Autodesk Inventor part; units mm, degrees
ref_plane "YZ Plane" through (0, 0, 0) normal (1, 0, 0) x (0, 1, 0)
ref_plane "XZ Plane" through (0, 0, 0) normal (0, 1, 0) x (-1, 0, 0)
ref_plane "XY Plane" through (0, 0, 0) normal (0, 0, 1) x (1, 0, 0)
sketch "Sketch1" plane through (0, 0, 0) normal (0, 0, 1) x (1, 0, 0)
  arc A0 (-13.7715, -6.45) -> (-16.2715, -6.45) centre (-15.0215, -6.45) ccw
  line L0 (-16.2715, -6.45) -> (-16.2715, -7.25)
  arc A1 (-17.2715, -8.25) -> (-16.2715, -7.25) centre (-17.2715, -7.25) ccw
  line L1 (-17.2715, -8.25) -> (-18.7715, -8.25)
  arc A2 (-19.7715, -7.25) -> (-18.7715, -8.25) centre (-18.7715, -7.25) ccw
  line L2 (-19.7715, -7.25) -> (-19.7715, 7.25)
  arc A3 (-18.7715, 8.25) -> (-19.7715, 7.25) centre (-18.7715, 7.25) ccw
  line L3 (-18.7715, 8.25) -> (-17.2715, 8.25)
  arc A4 (-16.2715, 7.25) -> (-17.2715, 8.25) centre (-17.2715, 7.25) ccw
  line L4 (-16.2715, 7.25) -> (-16.2715, 6.45)
  arc A5 (-16.2715, 6.45) -> (-13.7715, 6.45) centre (-15.0215, 6.45) ccw
  arc A6 (-13.5715, -6.45) -> (-16.4715, -6.45) centre (-15.0215, -6.45) ccw
  line L5 (-16.4715, -6.45) -> (-16.4715, -7.25)
  arc A7 (-17.2715, -8.05) -> (-16.4715, -7.25) centre (-17.2715, -7.25) ccw
  line L6 (-17.2715, -8.05) -> (-18.7715, -8.05)
  arc A8 (-19.5715, -7.25) -> (-18.7715, -8.05) centre (-18.7715, -7.25) ccw
  line L7 (-19.5715, -7.25) -> (-19.5715, 7.25)
  arc A9 (-18.7715, 8.05) -> (-19.5715, 7.25) centre (-18.7715, 7.25) ccw
  line L8 (-18.7715, 8.05) -> (-17.2715, 8.05)
  arc A10 (-16.4715, 7.25) -> (-17.2715, 8.05) centre (-17.2715, 7.25) ccw
  line L9 (-16.4715, 7.25) -> (-16.4715, 6.45)
  arc A11 (-16.4715, 6.45) -> (-13.5715, 6.45) centre (-15.0215, 6.45) ccw
  circle A12 centre (-5.5215, 0) radius 1.6
  circle A13 centre (7.4785, 5) radius 0.5969
  circle A14 centre (7.4785, -5) radius 0.5969
  line L10 (13.4965, -5.336) -> (13.0086, -5.8402)
  arc A15 (13.4965, -5.336) -> (1.4605, 5.336) centre (7.4785, 0) ccw
  line L11 (1.1785, 5) -> (1.4605, 5.336)
  line L12 (-15.5215, 5) -> (1.1785, 5)
  line L13 (-15.5215, -5) -> (-15.5215, 5)
  line L14 (1.1785, -5) -> (-15.5215, -5)
  arc A16 (1.1785, -5) -> (13.0086, -5.8402) centre (7.4785, 0) ccw
  arc A17 (-0.6485, -6.45) -> (-0.6486, 6.45) centre (7.4785, 0) ccw
  line L15 (-0.6485, -6.45) -> (-15.5215, -6.45)
  line L16 (-15.5215, -6.45) -> (-15.5215, 6.45)
  line L17 (-15.5215, 6.45) -> (-0.6486, 6.45)
  line L18 (7.4785, 0) -> (-0.6485, -6.45)
  line L19 (7.4785, 0) -> (-0.6486, 6.45)
  circle A18 centre (7.4785, 0) radius 8.243
  point P0 (0, 0)
  point P1 (-15.03, 5)
  point P2 (-15.5215, 5.0889)
  point P3 (-13.5715, 6.45)
  dimension "d0" = 0.2
  dimension "d1" = 0.2
extrude "Extrusion1" add sketch "Sketch1" against normal blind 10 contours A6 L14 A18 L18 L15 | L16 L14 A6 | A6 L5 A7 L6 A8 L7 A9 L8 A10 L9 A11 L16 L13 | L14 L13 L12 A18 | L18 A18 L19 A17 | L19 A18 L12 A11 L17 | A12
sketch "Sketch2" plane through (0, 0, 0) normal (0, 0, 1) x (1, 0, 0)
  circle A0 centre (-5.5215, 0) radius 1.6
  circle A1 centre (7.4785, 5) radius 0.5969
  circle A2 centre (7.4785, -5) radius 0.5969
  line L0 (13.4965, -5.336) -> (13.0086, -5.8402)
  arc A3 (13.4965, -5.336) -> (1.4605, 5.336) centre (7.4785, 0) ccw
  line L1 (1.1785, 5) -> (1.4605, 5.336)
  line L2 (-15.5215, 5) -> (1.1785, 5)
  line L3 (-15.5215, -5) -> (-15.5215, 5)
  line L4 (1.1785, -5) -> (-15.5215, -5)
  arc A4 (1.1785, -5) -> (13.0086, -5.8402) centre (7.4785, 0) ccw
  line L5 (-15.7215, 5.2) -> (1.0853, 5.2)
  line L6 (1.0853, 5.2) -> (1.309, 5.4667)
  arc A5 (13.6433, -5.472) -> (1.309, 5.4667) centre (7.4785, 0) ccw
  line L7 (13.6433, -5.472) -> (13.1493, -5.9824)
  arc A6 (1.0826, -5.2) -> (13.1493, -5.9824) centre (7.4785, 0) ccw
  line L8 (1.0826, -5.2) -> (-15.7215, -5.2)
  line L9 (-15.7215, -5.2) -> (-15.7215, 5.2)
  point P0 (0, 0)
  dimension "d4" = 0.2
extrude "Extrusion2" cut sketch "Sketch2" against normal blind 1.6 contours L0 A4 L4 L3 L2 L1 A3 | L5 L6 A5 L7 A6 L8 L9
sketch "Sketch3" plane through (-5.5215, 0, 0) normal (0, 0, 1) x (1, 0, 0)
  circle A0 centre (0, 0) radius 2
  point P0 (5.5215, 0)
  dimension "d7" = 4
extrude "Extrusion3" cut sketch "Sketch3" against normal blind 8
sketch "Sketch4" plane through (-19.5715, -7.25, 0) normal (-1, 0, 0) x (0, 0, 1)
  circle A0 centre (-5, 7.25) radius 2
  point P0 (0, 7.25)
  dimension "d10" = 4
  dimension "d11" = 5
extrude "Extrusion4" cut sketch "Sketch4" against normal blind 8
sketch "Sketch5" plane through (0, 0, 0) normal (0, 0, 1) x (1, 0, 0)
  line L0 (-13.7715, -9.5) -> (-13.7715, -6.45)
  line L1 (-13.7715, 6.45) -> (-13.7715, 9.5)
  line L2 (-13.7715, -9.5) -> (3.307, -9.5)
  arc A0 (-0.6485, -6.45) -> (-0.6486, 6.45) centre (7.4785, 0) ccw
  line L3 (-13.7715, 9.5) -> (3.307, 9.5)
  line L4 (-0.6485, -6.45) -> (-13.5715, -6.45)
  line L5 (-13.5715, -6.45) -> (-13.5715, -9.5)
  arc A1 (-15.03, 5) -> (-13.5715, 6.45) centre (-15.0215, 6.45) ccw
  line L6 (-13.5715, 6.45) -> (-13.5715, 9.5)
  line L7 (-0.6486, 6.45) -> (-13.5715, 6.45)
  point P0 (0, 0)
extrude "Extrusion5" add sketch "Sketch5" against normal up to surface (10 mm away)
fillet "Fillet2" radius 1 6 edges at (17.854, 0, 0) (-5.1322, -9.5, 0) (-5.1323, 9.5, 0) (17.854, 0, -10) (-5.1323, 9.5, -10) (-5.1322, -9.5, -10)
properties part number "TransducerPCB_Holder"
The listing builds one solid part. Answer for the finished solid, in the listing's coordinates (mm). A direction names the side the tool comes from. Give positions to 0.01 mm unless a question says otherwise; leave off trailing zeros. Loops run counter-clockwise (first coordinate to the right, second up) from the corner with the lowest first, then second, coordinate; pieces in that order, holes last. Notation, with made-up numbers: (79.25, 67) - (107.25, 67) arc R5 ccw to (107.25, 75) - close; hole circle Ø8 at (35, 64.25). An arc over 180 degrees is marked (long way). Return JSON: item names as keys, results as strings. Group by question number.
1. Find section C-C (z = -2.25). Write down the section's boundary in (x, y).
2. Straight lines are drawn through the part: line 1 (X direction, y = -5.25, z = -2.5); line 2 (X direction, y = -6.75, z = -1); line 3 (Z direction, x = -11, y = -2.75). For each, find the intervals that lie inside material, in ascending order. Write a range as [from, to].
3. Determine the mould class of faces 5 (the cylindrical face through (17.85, -0.29, -4.94)), 6 (the flat face through (-18, 0, 0)), 7 (the flat face through (-9, 0, -1.6)) for opening direction Y: pulls with the +Y half, pulls with the -Y half, needs draft (parallel to the pull), parting line crosses it, or undercut.
4. Find section B-B (x = -2.5). Write down the section's boundary in (y, z).
5. Which of the six approach directions +Z, -Z, +X, -X, +Y, -Y give full straight-line access (tool end or side, diameter ignored) to faces 1 (the cylindrical face through (-4.905, -9.215, -9.699)), 2 (the flat face through (-13.572, -8, -5)), 3 (the flat face through (-6, 0, -8)), 4 (the flat face through (-5, 9.5, -5))?
6. Given pin 1 Ø1.2 at (x, z) = (-18, -6) entering from +Y; pin 2 Ø1.6 at (x, z) = (-17.5, -3.5) entering from -Y; pin 3 Ø5 at (x, z) = (13.5, -3.5) entering from -Y, each flat-ended and moving along its own axis, determine where each tip first touches the part or whether it passes through.
7. Find section D-D (y = 6). State how many separate pieces and enclosed holes the cut face has, then the cut area to 3 significant figures.
8. Find section A-A (z = -5). Write down the section's boundary in (x, y), then the cut area to 3 significant figures.
Verdict:
{
 "1": {"outline": "(-19.57, -7.25) arc R0.8 ccw to (-18.77, -8.05) - (-17.27, -8.05) arc R0.8 ccw to (-16.47, -7.25) - (-16.47, -6.45) arc R1.45 cw to (-13.57, -6.45) - (-13.57, -9.5) - (3.31, -9.5) arc R10.38 ccw (long way) to (3.31, 9.5) - (-13.57, 9.5) - (-13.57, 6.45) arc R1.45 cw to (-15.02, 5) - (-15.52, 5) - (-15.52, 5.09) arc R1.45 cw to (-16.47, 6.45) - (-16.47, 7.25) arc R0.8 ccw to (-17.27, 8.05) - (-18.77, 8.05) arc R0.8 ccw to (-19.57, 7.25) - close; hole circle Ø4 at (-5.52, 0); hole circle Ø16.49 at (7.48, 0)"},
 "2": {"line 1": "x = [-19.57, -15.84], [-14.21, 1.12], [13.83, 16.43]", "line 2": "x = [-19.57, -16.47], [-13.57, 2.75], [12.21, 15.36]", "line 3": "z = [-10, -1.6]"},
 "3": {"face 5": "parting line crosses it", "face 6": "needs draft", "face 7": "undercut"},
 "4": {"outline": "(-9.5, -9) arc R1 ccw to (-8.5, -10) - (8.5, -10) arc R1 ccw to (9.5, -9) - (9.5, -1) arc R1 ccw to (8.5, 0) - (5.2, 0) - (5.2, -1.6) - (-5.2, -1.6) - (-5.2, 0) - (-8.5, 0) arc R1 ccw to (-9.5, -1) - close"},
 "5": {"face 1": "-Z, -X, -Y", "face 2": "+Z, -Z, -Y", "face 3": "+Z", "face 4": "+Z, -Z, -X, +Y"},
 "6": {"pin 1": "stops at y = 8.05", "pin 2": "stops at y = -8.05", "pin 3": "stops at y = -9.76"},
 "7": {"separate pieces": "3", "enclosed holes": "0", "area": "214 mm^2"},
 "8": {"outline": "(-19.57, -7.25) arc R0.8 ccw to (-18.77, -8.05) - (-17.27, -8.05) arc R0.8 ccw to (-16.47, -7.25) - (-16.47, -6.45) arc R1.45 cw to (-13.57, -6.45) - (-13.57, -9.5) - (3.31, -9.5) arc R10.38 ccw (long way) to (3.31, 9.5) - (-13.57, 9.5) - (-13.57, 6.45) arc R1.45 cw to (-15.02, 5) - (-15.52, 5) - (-15.52, 5.09) arc R1.45 cw to (-16.47, 6.45) - (-16.47, 7.25) arc R0.8 ccw to (-17.27, 8.05) - (-18.77, 8.05) arc R0.8 ccw to (-19.57, 7.25) - (-19.57, 2) - (-11.57, 2) - (-11.57, -2) - (-19.57, -2) - close; hole circle Ø4 at (-5.52, 0); hole circle Ø16.49 at (7.48, 0)", "area": "396 mm^2"}
}
